Work out the finished part from the listing and answer in its coordinate system (mm). A direction names the side the tool comes from. Give positions to 0.01 mm unless a question says otherwise; leave off trailing zeros. Order: outer loops, then holes, each group sorted by start corner. A loop starts at its lowest first (then second) coordinate and runs counter-clockwise, first axis right, second up. Notation, with made-up numbers: (59.5, 36.5) - (79.5, 36.5) arc R25 cw to (79.5, 66.5) - close; hole circle Ø4 at (-26.75, 80). An arc over 180 degrees is marked (long way). Write each question's results on one line, items separated by ' | '.
from build123d import *

# Parameters (mm, degrees)
F0_W     = 70
F0_H     = 35
F1_DEPTH = 35
F2_W     = 21
F2_H     = 19
F3_DEPTH = 26.5
F4_W     = 12.5
F4_H     = 12.5
F5_DEPTH = 10
F7_DEPTH = 12


with BuildPart() as f1:
    # F0 (on Top) → F1 (new body)
    with BuildSketch(Plane.XY):
        Rectangle(F0_W, F0_H)
    extrude(amount=F1_DEPTH)

    # F2 (on Right) → F3 (cut, symmetric)
    with BuildSketch(Plane.YZ):
        with Locations((0, 17.5)):
            Rectangle(F2_W, F2_H)
    extrude(amount=F3_DEPTH, both=True, mode=Mode.SUBTRACT)

    # F4 (on face) → F5 (cut)
    with BuildSketch(Plane.YZ.offset(35)):
        with Locations((0, 17.5)):
            Rectangle(F4_W, F4_H)
    extrude(amount=-F5_DEPTH, mode=Mode.SUBTRACT)

    # F6 (on face) → F7 (cut)
    with BuildSketch(Plane.XY.offset(35)):
        Polygon((26.5, 10.5), (-26.5, 10.5), (-26.5, -10.5), (26.5, -10.5), (26.5, -6.25), (35, -6.25), (35, 6.25), (26.5, 6.25), align=None)
    extrude(amount=-F7_DEPTH, mode=Mode.SUBTRACT)


solid = f1.part
1. A cutting plane is placed at B-B, the plane x = 5.5. Write down the section's boundary in (y, z).
Answer list:
outline: (-17.5, 0) - (17.5, 0) - (17.5, 35) - (10.5, 35) - (10.5, 8) - (-10.5, 8) - (-10.5, 35) - (-17.5, 35) - close
2. Given P1, Ø6, axis at y = -2, z = 24, coming from the +X side; P2, Ø2, axis at x = -6.5, y = -1, coming from the +Z side; P3, Ø2.5, axis at x = 32.5, y = -2, coming from the +Z side, each flat-ended and moving along its own axis, determine where each tip first touches the part or whether it passes through.
Answer list:
P1: x = -26.5 | P2: z = 8 | P3: z = 11.25
3. A cutting plane is placed at A-A, the plane z = 10.5. Write down the section's boundary in (x, y), then the cut area to 3 significant figures.
Answer list:
outline: (-35, -17.5) - (35, -17.5) - (35, 17.5) - (-35, 17.5) - close; hole (-26.5, -10.5) - (26.5, -10.5) - (26.5, 10.5) - (-26.5, 10.5) - close | area: 1,340 mm^2
4. Determine the mould class of faces 4 (the face through (-26.5, 0, 22)), 5 (the face through (-35, 0, 17)), 6 (the face through (0, 12, 35)) for opening direction X: +X half, -X half, draft (parallel to the pull), parting line (faces both ways), or undercut.
Answer list:
face 4: undercut | face 5: -X half | face 6: draft
5. A cutting plane is placed at D-D, the plane z = 23.5. Write down the section's boundary in (x, y), then the cut area to 3 significant figures.
Answer list:
outline: (-35, -17.5) - (35, -17.5) - (35, -6.25) - (26.5, -6.25) - (26.5, -10.5) - (-26.5, -10.5) - (-26.5, 10.5) - (26.5, 10.5) - (26.5, 6.25) - (35, 6.25) - (35, 17.5) - (-35, 17.5) - close | area: 1,230 mm^2
6. Straight lines are drawn through the part: line 1 (X direction, y = -3, z = 11); line 2 (Y direction, x = -8, z = 33); line 3 (Y direction, x = 28.5, z = 19). For each, find the intervals that lie inside material, in ascending order. Write a range as [from, to].
Answer list:
line 1: [-35, -26.5], [26.5, 35] | line 2: [-17.5, -10.5], [10.5, 17.5] | line 3: [-17.5, -6.25], [6.25, 17.5]
7. A cutting plane is placed at C-C, the plane y = -5. Write down the section's boundary in (x, z).
Answer list:
outline: (-35, 0) - (35, 0) - (35, 11.25) - (26.5, 11.25) - (26.5, 8) - (-26.5, 8) - (-26.5, 35) - (-35, 35) - close
8. A tool of negligible diameter and unlimited length cuts with its end or side. For faces 1 (the face through (0, 0, 8)), 2 (the face through (31, 6.25, 23)), 3 (the face through (0, -17.5, 17)), from which of +Z, -Z, +X, -X, +Y, -Y can it reach the whole face along a straight path? Write none if from no direction.
Answer list:
face 1: +Z | face 2: +Z, +X | face 3: +Z, -Z, +X, -X, -Y
